from build123d import *

# Parameters (mm, degrees)
CROQUIS1_R              = 5
SALIENTE_EXTRUIR1_DEPTH = 20
CROQUIS2_W              = 100
CROQUIS2_H              = 30
SALIENTE_EXTRUIR2_DEPTH = 100
CROQUIS3_W              = 100
CROQUIS3_H              = 10
CORTAR_EXTRUIR1_DEPTH   = 80


with BuildPart() as part:
    # Croquis1 → Saliente-Extruir1 (new body)
    with BuildSketch(Plane(origin=(0, 0, 0), x_dir=(1, 0, 0), z_dir=(0, 1, 0))):
        with BuildLine():
            Line((63.639610307, 21.213203436), (-21.213203436, -63.639610307))
            ThreePointArc((-21.213203436, -63.639610307), (-63.639610307, -63.639610307), (-63.639610307, -21.213203436))
            Line((-63.639610307, -21.213203436), (21.213203436, 63.639610307))
            ThreePointArc((21.213203436, 63.639610307), (63.639610307, 63.639610307), (63.639610307, 21.213203436))
        make_face()
        with Locations(Location((-42.426406871, -42.426406871, 0), (0, 0, 270))):
            Circle(CROQUIS1_R, mode=Mode.SUBTRACT)
        with Locations(Location((42.426406871, 42.426406871, 0), (0, 0, 90))):
            Circle(CROQUIS1_R, mode=Mode.SUBTRACT)
    extrude(amount=SALIENTE_EXTRUIR1_DEPTH)

    # Croquis2 → Saliente-Extruir2 (add)
    with BuildSketch(Plane.XZ):
        Rectangle(CROQUIS2_W, CROQUIS2_H)
    extrude(amount=SALIENTE_EXTRUIR2_DEPTH)

    # Croquis3 → Cortar-Extruir1 (cut)
    with BuildSketch(Plane.XZ.offset(100)):
        Rectangle(CROQUIS3_W, CROQUIS3_H)
    extrude(amount=-CORTAR_EXTRUIR1_DEPTH, mode=Mode.SUBTRACT)


solid = part.part
Check sheet for the modelled part. Datum: model origin and axes. Units: mm. A direction names the side the tool comes from. Round coordinates to 2 decimals unless told otherwise and drop trailing zeros. Loops run counter-clockwise (first coordinate to the right, second up) from the corner with the lowest first, then second, coordinate; pieces in that order, holes last.
1. Sectioned sample at D-D on z = -11.5. Record the boundary of the cut face in (x, y), and give its area (3 significant figures).
2. Sectioned sample at A-A on y = -51. Record the boundary of the cut face in (x, z), and give its area (3 significant figures).
3. Sectioned sample at B-B on z = -42. Record the boundary of the cut face in (x, y), and give its area (3 significant figures).
4. Mould release check, pull along Z, two halves, no side actions. Record for faces 1 (the flat face through (-21.807, 9.86, -20.619)), 2 (the flat face through (-44, 0, -9)), 3 (the cylindrical face through (-40.925, 9.86, 47.196)): released by +Z, released by -Z, zero draft, split by the parting line, or undercut.
5. Sectioned sample at C-C on x = 44.5. Record the boundary of the cut face in (y, z).
6. Gauge pin test, flat ends, axial feed: pin 1 Ø4 at (x, y) = (-13, -5) entering from +Z; pin 2 Ø1.5 at (y, z) = (6.5, -15) entering from -X; pin 3 Ø13 at (x, z) = (42.43, -42.43) entering from +Y; pin 4 Ø3 at (x, z) = (16, 1.5) entering from -Y. Record the tip position at first contact, or that the pin passes through.
7. Scan lines: probe 1 along Z at (x, y) = (-11, -24.5); probe 2 along Z at (x, y) = (-11.5, -18.5); probe 3 along Y at (x, z) = (10, -52). Record each from-to range of solid material in increasing order.
8. Set-up check for faces 4 (the flat face through (-50, -49, -7)), 5 (the flat face through (44, 0, 9)), 6 (the flat face through (50, -49, -7)): record each of +Z, -Z, +X, -X, +Y, -Y from which the full face is reachable in a straight line by a thin tool's end or side.
Recorded:
1. outline: (-50, -100) - (50, -100) - (50, 0) - (53.93, 0) - (53.93, 20) - (-30.93, 20) - (-30.93, 0) - (-50, 0) - close
1. area: 11,700 mm2
2. outline: (-50, -15) - (50, -15) - (50, -5) - (-50, -5) - close; (-50, 5) - (50, 5) - (50, 15) - (-50, 15) - close
2. area: 2,000 mm2
3. outline: (-0.43, 0) - (37.44, 0) - (37.44, 20) - (-0.43, 20) - close; (47.41, 0) - (72.42, 0) - (72.42, 20) - (47.41, 20) - close
3. area: 1,260 mm2
4. face 1: released by -Z
4. face 2: zero draft
4. face 3: undercut
5. outline: (-100, -15) - (0, -15) - (0, -37.88) - (20, -37.88) - (20, -2.07) - (0, -2.07) - (0, 15) - (-100, 15) - (-100, 5) - (-20, 5) - (-20, -5) - (-100, -5) - close; (0, -72.35) - (20, -72.35) - (20, -46.98) - (0, -46.98) - close
6. pin 1: stops at z = 15
6. pin 2: stops at x = -28.18
6. pin 3: stops at y = 20
6. pin 4: stops at y = -20
7. probe 1: z = -15 to -5, 5 to 15
7. probe 2: z = -15 to 15
7. probe 3: y = 0 to 20
8. face 4: +Z, -Z, -X, -Y
8. face 5: +Z, +X, +Y
8. face 6: +Z, -Z, +X, -Y
